Answer from the drawing. Dimensions are ordinates in mm from the lowest x, y and z of the part. Round coordinates to 2 decimals unless told otherwise and drop trailing zeros. Order: outer loops, then holes, each group sorted by start corner. A loop starts at its lowest first (then second) coordinate and runs counter-clockwise, first axis right, second up.
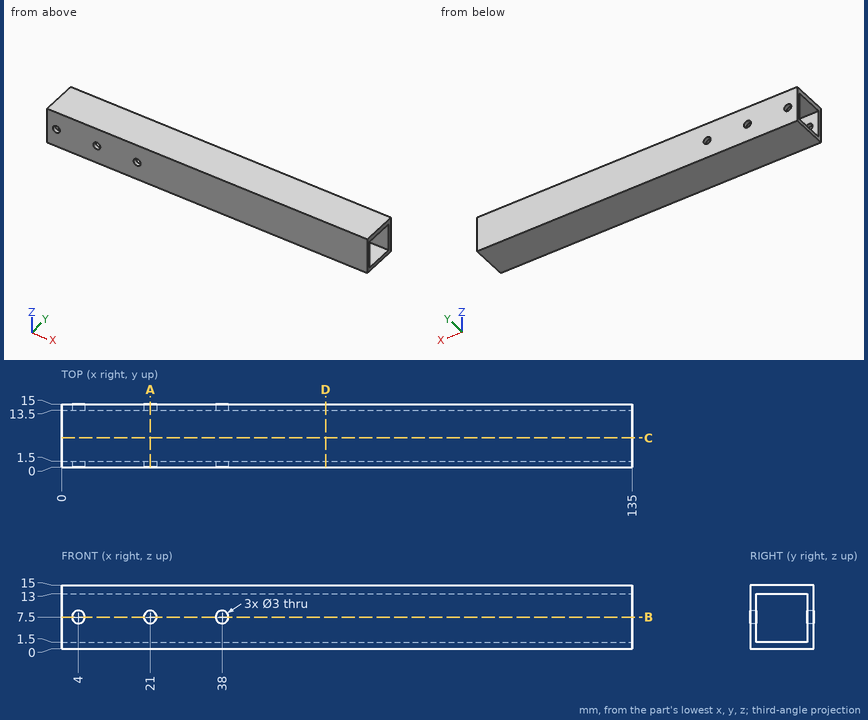
Q1. A flat-ended cylindrical pin translates along its axis: pin 1 (2.5 mm diameter, centred on x = 21, z = 7.5, fed in from -Y). Find the tip coordinate at first contact, or state that the pin passes through.
Outcome:
pin 1: passes through
Q2. A cutting plane is placed at D-D, the plane x = 62.5. Give the vertices of the cut face in (y, z), plus the area to 3 significant figures.
Outcome:
outline: (0, 0) - (15, 0) - (15, 15) - (0, 15) - close; hole (1.5, 1.5) - (13.5, 1.5) - (13.5, 13) - (1.5, 13) - close
area: 87.0 mm2
Q3. A cutting plane is placed at C-C, the plane y = 7. Give the vertices of the cut face in (x, z), plus the area to 4 significant figures.
Outcome:
outline: (0, 0) - (135, 0) - (135, 1.5) - (0, 1.5) - close; (0, 13) - (135, 13) - (135, 15) - (0, 15) - close
area: 472.5 mm2
Q4. A cutting plane is placed at A-A, the plane x = 21. Give the vertices of the cut face in (y, z).
Outcome:
outline: (0, 0) - (15, 0) - (15, 6) - (13.5, 6) - (13.5, 1.5) - (1.5, 1.5) - (1.5, 6) - (0, 6) - close; (0, 9) - (1.5, 9) - (1.5, 13) - (13.5, 13) - (13.5, 9) - (15, 9) - (15, 15) - (0, 15) - close
Q5. A cutting plane is placed at B-B, the plane z = 7.5. Give the number of separate pieces and of enclosed holes in the cut face, plus the area to 3 significant figures.
Outcome:
separate pieces: 8
enclosed holes: 0
area: 378 mm2
Q6. Straight lines are drawn through the part: probe 1 along X at (y, z) = (14.5, 7.5); probe 2 along Y at (x, z) = (107.5, 3.75); probe 3 along Z at (x, y) = (40, 10.5). For each, find the intervals that lie inside material, in ascending order.
Outcome:
probe 1: x = 0 to 2.5, 5.5 to 19.5, 22.5 to 36.5, 39.5 to 135
probe 2: y = 0 to 1.5, 13.5 to 15
probe 3: z = 0 to 1.5, 13 to 15
